Source: CAD feature listing. Evaluate the final solid. Frame: model axes, mm. A direction names the side the tool comes from. Give positions to 0.01 mm unless a question says otherwise; leave off trailing zeros. Order: outer loops, then holes, each group sorted by start corner. A loop starts at its lowest first (then second) coordinate and runs counter-clockwise, first axis right, second up. Notation, with made-up numbers: (3.25, -28) - (10.25, -28) arc R29 ccw to (10.25, 2) - close; hole circle Ø5 at (48, 56.5). An arc over 180 degrees is marked (long way). Answer as CSV lines item,"result".
```python
from build123d import *

# Parameters (mm, degrees)
BOX009_W               = 20.4
BOX009_H               = 25.4
BOX009_DEPTH           = 10
BOX008_W               = 26.9
BOX008_H               = 26
BOX008_DEPTH           = 25.4
BOX007_W               = 30.9
BOX007_H               = 5.4
BOX007_DEPTH           = 30.4
CUT004_PITCH_ANGLE     = -90
CUT004_PLACEMENT_ANGLE = 90
BOX_W                  = 25.4
BOX_H                  = 30.4
BOX_DEPTH              = 2
BOX003_W               = 25.4
BOX003_H               = 2
BOX003_DEPTH           = 5
BOX002_W               = 25.4
BOX002_H               = 2
BOX002_DEPTH           = 5
BOX004_W               = 17
BOX004_H               = 10
BOX004_DEPTH           = 4
CYLINDER_R             = 5
CYLINDER_DEPTH         = 4
BOX001_W               = 25.4
BOX001_H               = 30.4
BOX001_DEPTH           = 2


with BuildPart() as gap:
    # Box009 → Box009 (new body)
    with BuildSketch(Plane(origin=(5, 0, 0), x_dir=(1, 0, 0), z_dir=(0, 0, 1))):
        with Locations((10.2, 12.7)):
            Rectangle(BOX009_W, BOX009_H)
    extrude(amount=BOX009_DEPTH)


with BuildPart() as bar:
    # Box008 → Box008 (new body)
    with BuildSketch(Plane(origin=(2, 0, 2.5), x_dir=(1, 0, 0), z_dir=(0, 0, 1))):
        with Locations((13.45, 13)):
            Rectangle(BOX008_W, BOX008_H)
    extrude(amount=BOX008_DEPTH)


with BuildPart() as clip:
    # Box007 → Box007 (new body)
    with BuildSketch(Plane.XY):
        with Locations((15.45, 2.7)):
            Rectangle(BOX007_W, BOX007_H)
    extrude(amount=BOX007_DEPTH)

    # Cut003: cut Bar
    add(bar.part, mode=Mode.SUBTRACT)

    # Cut004: cut Gap
    add(gap.part, mode=Mode.SUBTRACT)


with BuildPart() as clip_1:
    # Cut004 pitch: moved
    add(clip.part.rotate(Axis((0, 0, 0), (0, 1, 0)), CUT004_PITCH_ANGLE))


with BuildPart() as clip_2:
    # Cut004 placement: moved
    add(clip_1.part.moved(Location((5.4, 30.4, 9))).rotate(Axis((5.4, 30.4, 9), (0, 0, 1)), CUT004_PLACEMENT_ANGLE))


with BuildPart() as top:
    # Box → Box (new body)
    with BuildSketch(Plane.XY.offset(7)):
        with Locations((12.7, 15.2)):
            Rectangle(BOX_W, BOX_H)
    extrude(amount=BOX_DEPTH)


with BuildPart() as right:
    # Box003 → Box003 (new body)
    with BuildSketch(Plane(origin=(0, 28.4, 2), x_dir=(1, 0, 0), z_dir=(0, 0, 1))):
        with Locations((12.7, 1)):
            Rectangle(BOX003_W, BOX003_H)
    extrude(amount=BOX003_DEPTH)


with BuildPart() as left:
    # Box002 → Box002 (new body)
    with BuildSketch(Plane.XY.offset(2)):
        with Locations((12.7, 1)):
            Rectangle(BOX002_W, BOX002_H)
    extrude(amount=BOX002_DEPTH)


with BuildPart() as cube:
    # Box004 → Box004 (new body)
    with BuildSketch(Plane(origin=(9, 11.2, 9), x_dir=(1, 0, 0), z_dir=(0, 0, 1))):
        with Locations((8.5, 5)):
            Rectangle(BOX004_W, BOX004_H)
    extrude(amount=BOX004_DEPTH)


with BuildPart() as cylinder:
    # Cylinder → Cylinder (new body)
    with BuildSketch(Plane(origin=(9, 16.2, 9), x_dir=(1, 0, 0), z_dir=(0, 0, 1))):
        Circle(CYLINDER_R)
    extrude(amount=CYLINDER_DEPTH)


with BuildPart() as fusion003:
    # Box001 → Box001 (new body)
    with BuildSketch(Plane.XY.offset(10)):
        with Locations((12.7, 15.2)):
            Rectangle(BOX001_W, BOX001_H)
    extrude(amount=BOX001_DEPTH)

    # Cut: cut Cylinder
    add(cylinder.part, mode=Mode.SUBTRACT)

    # Cut001: cut Cube
    add(cube.part, mode=Mode.SUBTRACT)


with BuildPart() as fusion003_1:
    # Cut001 placement: moved
    add(fusion003.part.moved(Location((0, 0, -10))))

    # Fusion: union Left
    add(left.part)

    # Fusion001: union Right
    add(right.part)

    # Fusion002: union Top
    add(top.part)

    # Fusion003: union Clip
    add(clip_2.part)


solid = fusion003_1.part
```
(1) Cut plane D-D (z = 29). Return loops of the section in (x, y), then the cut area to 3 significant figures.
Completed:
outline,"(0, 0) - (5.4, 0) - (5.4, 2.5) - (0, 2.5) - close"
area,"13.5 mm²"
(2) Ray query, line 1 (Z direction, x = 2.25, y = 22); line 2 (Z direction, x = 14.25, y = 9); line 3 (Y direction, x = 4.5, z = 5). Return the intervals inside material, ascending. Write a range as from..to.
Completed:
line 1,"0..2, 7..11, 37.9..39.9"
line 2,"0..2, 7..9"
line 3,"0..2, 28.4..30.4"
(3) Contact query for flat-ended pins moving along their axis: pin 1 (6 mm diameter, centred on x = 2, z = 27, fed in from +Y); pin 2 (6 mm diameter, centred on y = 17, z = 35, fed in from +X); pin 3 (8 mm diameter, centred on x = 22.5, y = 15.5, fed in from +Z). Output: stop coordinate, or through.
Completed:
pin 1,"y = 2.5"
pin 2,"x = 5.4"
pin 3,"z = 9"
(4) Cut plane A-A (y = 24.5). Return loops of the section in (x, z), then the cut area to 3 significant figures.
Completed:
outline,"(0, 0) - (25.4, 0) - (25.4, 2) - (0, 2) - close; (0, 7) - (25.4, 7) - (25.4, 9) - (5.4, 9) - (5.4, 11) - (0, 11) - close; (0, 37.9) - (5.4, 37.9) - (5.4, 39.9) - (0, 39.9) - close"
area,"123 mm²"
(5) Mould query, pull axis Z, two halves, no side actions, for faces 1 (the flat face through (0, 13, 10)), 2 (the flat face through (13, 9, 0)), 3 (the flat face through (13, 2, 4)), 4 (the flat face through (13, 28.4, 4)). Classes: released by +Z, released by -Z, zero draft, split by the parting line, or undercut.
Completed:
face 1,"zero draft"
face 2,"released by -Z"
face 3,"undercut"
face 4,"undercut"
(6) Access query for faces 5 (the flat face through (17, 11.2, 1)), 6 (the flat face through (15, 15, 9)), 7 (the flat face through (3, 29, 34.4)), 8 (the flat face through (13, 15, 7)). Directions: +Z, -Z, +X, -X, +Y, -Y. A direction counts if a zero-diameter tool reaches every point of the face in a straight line with its end or side. Return the directions, or none.
Completed:
face 5,"-Z, +X"
face 6,"+Z, +X, +Y, -Y"
face 7,"+X, -X, +Y"
face 8,"+X, -X"
(7) Cut plane C-C (y = 16.2). Return loops of the section in (x, z).
Completed:
outline,"(0, 0) - (4, 0) - (4, 2) - (0, 2) - close; (0, 7) - (25.4, 7) - (25.4, 9) - (5.4, 9) - (5.4, 11) - (0, 11) - close; (0, 37.9) - (5.4, 37.9) - (5.4, 39.9) - (0, 39.9) - close"
(8) Cut plane B-B (x = 21.25). Return loops of the section in (y, z), then the cut area to 3 significant figures.
Completed:
outline,"(0, 0) - (11.2, 0) - (11.2, 2) - (2, 2) - (2, 7) - (28.4, 7) - (28.4, 2) - (21.2, 2) - (21.2, 0) - (30.4, 0) - (30.4, 9) - (0, 9) - close"
area,"122 mm²"
